from build123d import *

# Parameters (mm, degrees)
SKETCH1_R                = 25
BOSS_EXTRUDE1_DEPTH      = 3
BOSS_EXTRUDE2_DEPTH      = 10
BOSS_EXTRUDE2_DEPTH_BACK = 10
BOSS_EXTRUDE3_REACH      = 58.223
BOSS_EXTRUDE3_END_RADIUS = 25
SKETCH3_W                = 20
SKETCH3_H                = 3
SKETCH6_R                = 1
CUT_EXTRUDE1_DEPTH       = 20
CUT_EXTRUDE2_START       = -5
CUT_EXTRUDE2_DEPTH       = 5
LPATTERN1_COUNT          = 2
LPATTERN1_PITCH          = 10


with BuildPart() as part:
    # Sketch1 → Boss-Extrude1 (new body)
    with BuildSketch(Plane(origin=(0, 0, 0), x_dir=(1, 0, 0), z_dir=(0, 1, 0))):
        with Locations(Location((0, 0, 0), (0, 0, 270))):
            Circle(SKETCH1_R)
    extrude(amount=BOSS_EXTRUDE1_DEPTH)



with BuildPart() as body_2:
    # Sketch2 → Boss-Extrude2 (new, two sides: drawn at the far end of the back side and taken through both)
    with BuildSketch(Plane.XY.offset(-BOSS_EXTRUDE2_DEPTH_BACK)):
        with BuildLine():
            Line((25, 3), (25, 4))
            ThreePointArc((25, 4), (28.414213562, 5.414213562), (27, 2))
            Line((27, 2), (25, 0))
            Line((25, 0), (25, 3))
        make_face()
    extrude(amount=BOSS_EXTRUDE2_DEPTH + BOSS_EXTRUDE2_DEPTH_BACK)


with BuildPart() as part_1:
    add(part.part)

    add(body_2.part)  # Boss-Extrude3 merges body 2
    # Boss-Extrude3: up to this cylinder (the profile starts outside it)
    boss_extrude3_end = Plane(origin=(0, 1.5, 0), z_dir=(0, -1, 0)) * Cylinder(BOSS_EXTRUDE3_END_RADIUS, 167.446, mode=Mode.PRIVATE)
    # Sketch3 → Boss-Extrude3 (add, up to the surface)
    with BuildSketch(Plane.ZY.offset(-25), mode=Mode.PRIVATE) as boss_extrude3_sk1:
        with Locations((0, 1.5)):
            Rectangle(SKETCH3_W, SKETCH3_H)
    boss_extrude3_tool1 = extrude(boss_extrude3_sk1.sketch, amount=BOSS_EXTRUDE3_REACH, mode=Mode.PRIVATE) - boss_extrude3_end
    add(boss_extrude3_tool1.solids().sort_by_distance((25, 1.5, 0))[0])
    add(boss_extrude3_tool1.solids().sort_by_distance((25, 1.5, 0))[1])

    # Sketch6 → Cut-Extrude1 (cut)
    with BuildSketch(Plane.XY.offset(10)):
        with Locations((27, 4)):
            Circle(SKETCH6_R)
    extrude(amount=-CUT_EXTRUDE1_DEPTH, mode=Mode.SUBTRACT)

    # Sketch7 → Cut-Extrude2 (cut)
    with BuildSketch(Plane.XY.offset(10).offset(CUT_EXTRUDE2_START)):
        with BuildLine():
            Line((25, 3), (25.267949192, 3))
            ThreePointArc((25.267949192, 3), (28.931851653, 4.51763809), (25, 4))
            Line((25, 4), (25, 3))
        make_face()
    cut_extrude2 = extrude(amount=CUT_EXTRUDE2_DEPTH, mode=Mode.SUBTRACT)

    # LPattern1: Cut-Extrude2 ×2
    with Locations(*[(0, 0, -i * LPATTERN1_PITCH) for i in range(1, LPATTERN1_COUNT)]):
        add(cut_extrude2, mode=Mode.SUBTRACT)


solid = part_1.part
Model file for the job. Use its own axes, mm. A direction names the side the tool comes from. Round coordinates to 2 decimals unless told otherwise and drop trailing zeros. Loops run counter-clockwise (first coordinate to the right, second up) from the corner with the lowest first, then second, coordinate; pieces in that order, holes last. Notation, with made-up numbers: (89, 53) -> (138, 53) arc R10 cw to (138, 69) -> close; hole circle Ø7 at (-13, 11). An arc over 180 degrees is marked (long way). Answer as CSV lines item,"result". Start each with the question number.
1) Mould opens along Y. For faces 1 (the face through (25.987, 2.275, 7.465)), 2 (the face through (26, 3, 0)), 3 (the face through (26.263, 4.676, -7.465)) say: +Y half, -Y half, draft (parallel to the pull), parting line (faces both ways), or undercut.
2) Slice it at A-A (x = 0). List the corners of the cut face in (y, z), plus the area to 3 significant figures.
3) Probe line 1 along Z through (x, y) = (26.5, 2.8); line 2 along Y through (x, z) = (22.5, 3); line 3 along Z through (x, y) = (-10, 1.2). List the from-to ranges inside material, lowest first.
4) Pin check, flat tips, straight feed: P1, Ø12, axis at x = -10.5, z = 13, coming from the +Y side; P2, Ø2, axis at x = 27.5, y = 5, coming from the +Z side; P3, Ø2.5, axis at x = 27, y = 4, coming from the -Z side; P4, Ø1.5, axis at x = -19.5, y = 4.5, coming from the -Z side. Stop position of each tip, or through.
5) Tool access for faces 4 (the face through (26, 3, 5)), 5 (the face through (25.987, 2.275, -2.535)), 6 (the face through (25, 1, 10)), 7 (the face through (26, 3, -10)): list every direction of +Z, -Z, +X, -X, +Y, -Y with a clear straight run to the whole face (end or side of a thin tool).
6) Slice it at B-B (y = 1.05). List the corners of the cut face in (x, z), plus the area to 3 significant figures.
Filled in:
1,face 1,"+Y half"
1,face 2,"draft"
1,face 3,"undercut"
2,outline,"(0, -25) -> (3, -25) -> (3, 25) -> (0, 25) -> close"
2,area,"150 mm2"
3,line 1,"z = -10 to -5, 0 to 5"
3,line 2,"y = 0 to 3"
3,line 3,"z = -22.91 to 22.91"
4,P1,"stops at y = 3"
4,P2,"stops at z = 5"
4,P3,"stops at z = -10"
4,P4,"passes through"
5,face 4,"+Z, +X, +Y"
5,face 5,"+X, +Y"
5,face 6,"+Z, +X, +Y, -Y"
5,face 7,"-Z, +X, +Y, -Y"
6,outline,"(22.91, -10) -> (26.05, -10) -> (26.05, 10) -> (22.91, 10) arc R25 ccw (long way) to start"
6,area,"2,000 mm2"
